Could you check a few things on this model? Use its own coordinates, in mm. Coordinates: 2 decimals unless noted, no trailing zeros. Loops run counter-clockwise (first coordinate to the right, second up) from the corner with the lowest first, then second, coordinate; pieces in that order, holes last.
1) If I drill on line 1 along Z through (x, y) = (6, -0.5); line 2 along X through (y, z) = (-3, 0); line 3 along Z through (x, y) = (6, -2.5), over which ranges is the centre line in solid material (lowest first)?
2) Imagine slicing it at D-D on x = 38.5. Please give me the cut outline in (y, z), plus the area to 3 significant figures.
3) Imagine slicing it at C-C on x = 6. Please give me the cut outline in (y, z).
4) Imagine slicing it at A-A on z = 0. Please give me the cut outline in (x, y).
5) Imagine slicing it at B-B on y = 0. Please give me the cut outline in (x, z), plus the area to 3 significant figures.
6) Will these pins go through, and if not, where does the flat tip stop? P1, Ø1, axis at x = 36, y = 2.5, coming from the +Z side; P2, Ø4, axis at x = 31, y = 7, coming from the -Z side; P3, Ø1, axis at x = 54.5, y = -1, coming from the +Z side.
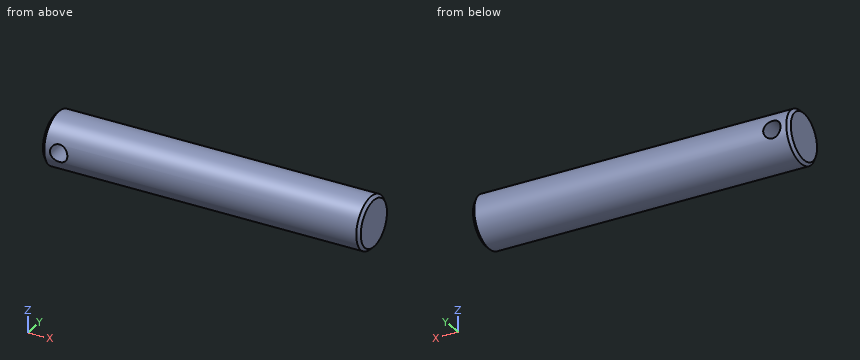
```python
from build123d import *

# Parameters (mm, degrees)
F0_R     = 9
F1_DEPTH = 110
F2_SIZE  = 1
F3_R     = 3
F4_DEPTH = 9


with BuildPart() as f1:
    # F0 (on Right) → F1 (new body)
    with BuildSketch(Plane.YZ):
        Circle(F0_R)
    extrude(amount=F1_DEPTH)

    # F2
    f2_edges = [f1.edges().sort_by_distance(p)[0] for p in [
        (110, -9, 0),
        (0, -9, 0),
    ]]
    chamfer(f2_edges, length=F2_SIZE)

    # F3 (on Front) → F4 (cut, symmetric)
    with BuildSketch(Plane.XZ):
        with Locations((6, 0)):
            Circle(F3_R)
    extrude(amount=F4_DEPTH, both=True, mode=Mode.SUBTRACT)


solid = f1.part
```
Filled in:
1. line 1: z = -8.99 to -3, 3 to 8.99
1. line 2: x = 0 to 3, 9 to 110
1. line 3: z = -8.65 to -3, 3 to 8.65
2. outline: circle Ø18 at (0, 0)
2. area: 254 mm2
3. outline: (-8.49, -3) arc R9 ccw to (8.49, -3) - close; (-8.49, 3) - (8.49, 3) arc R9 ccw to start
4. outline: (0, -8) - (1, -9) - (3, -9) - (3, 9) - (1, 9) - (0, 8) - close; (9, -9) - (109, -9) - (110, -8) - (110, 8) - (109, 9) - (9, 9) - close
5. outline: (0, -8) - (1, -9) - (109, -9) - (110, -8) - (110, 8) - (109, 9) - (1, 9) - (0, 8) - close; hole circle Ø6 at (6, 0)
5. area: 1,950 mm2
6. P1: stops at z = 8.77
6. P2: stops at z = -7.48
6. P3: stops at z = 8.99
